Source: CAD feature listing. Evaluate the final solid. Frame: model axes, mm. Coordinates: 2 decimals unless noted, no trailing zeros. Loops run counter-clockwise (first coordinate to the right, second up) from the corner with the lowest first, then second, coordinate; pieces in that order, holes last.
from build123d import *

# Parameters (mm, degrees)
F0_R     = 10
F1_DEPTH = 30
F3_D     = 10
F4_SIZE  = 1


with BuildPart() as f1:
    # F0 (on Top) → F1 (new body)
    with BuildSketch(Plane.XY):
        Circle(F0_R)
    extrude(amount=F1_DEPTH)

    # F3 (through all)
    with Locations(Plane(origin=(0, 0, 0), x_dir=(1, 0, 0), z_dir=(0, 0, -1))):
        with Locations((0, 0)):
            Hole(F3_D / 2)

    # F4
    f4_edges = [f1.edges().sort_by_distance(p)[0] for p in [
        (10, 0, 15),
        (-10, 0, 0),
        (-10, 0, 30),
        (-5, 0, 0),
        (-5, 0, 30),
    ]]
    chamfer(f4_edges, length=F4_SIZE)


solid = f1.part
Q1. Section C-C, the plane z = 9. Return the cut outline in (x, y).
Q2. Contact query for flat-ended pins moving along their axis: pin 1 Ø1 at (y, z) = (7.5, 16) entering from -X; pin 2 Ø10 at (x, z) = (4, 12.5) entering from +Y; pin 3 Ø11.5 at (x, y) = (0, 0) entering from -Z; pin 4 Ø3 at (y, z) = (7, 24.5) entering from +X. Output: stop coordinate, or through.
Q3. Draft query along X for faces 1 (the cylindrical face through (-2.17, -9.76, 14.8)), 2 (the flat face through (2, -6, 30)), 3 (the cylindrical face through (1.08, 4.88, 15.2)). Return one class per face: +X half, -X half, draft (parallel to the pull), parting line (faces both ways), or undercut.
Q4. Section A-A, the plane x = 0. Return the cut outline in (y, z).
Q5. Line query: line 1 along Y through (x, z) = (0, 17.75); line 2 along Y through (x, z) = (-4.25, 6); line 3 along X through (y, z) = (2.25, 19.5). Output: solid intervals per line, ascending.
Derived:
1. outline: circle Ø20 at (0, 0); hole circle Ø10 at (0, 0)
2. pin 1: stops at x = -7.14
2. pin 2: stops at y = 10
2. pin 3: stops at z = 0.25
2. pin 4: stops at x = 8.35
3. face 1: parting line
3. face 2: draft
3. face 3: undercut
4. outline: (-10, 1) - (-9, 0) - (-6, 0) - (-5, 1) - (-5, 29) - (-6, 30) - (-9, 30) - (-10, 29) - close; (5, 1) - (6, 0) - (9, 0) - (10, 1) - (10, 29) - (9, 30) - (6, 30) - (5, 29) - close
5. line 1: y = -10 to -5, 5 to 10
5. line 2: y = -9.05 to -2.63, 2.63 to 9.05
5. line 3: x = -9.74 to -4.47, 4.47 to 9.74
